from build123d import *

# Parameters (mm, degrees)
SKETCH1_R           = 18.5
BOSS_EXTRUDE1_DEPTH = 8.7
CUT_EXTRUDE1_START  = -5.7
SKETCH2_R           = 18.5
SKETCH2_R_2         = 17
CUT_EXTRUDE1_DEPTH  = 5.7
SKETCH3_R           = 14.2
CUT_EXTRUDE2_DEPTH  = 5.6
SKETCH4_R           = 4
BOSS_EXTRUDE2_DEPTH = 10
CHAMFER1_SIZE       = 2
SKETCH5_R           = 1.5
CUT_EXTRUDE3_DEPTH  = 30.259357478


with BuildPart() as part:
    # Sketch1 → Boss-Extrude1 (new body)
    with BuildSketch(Plane(origin=(0, 0, 0), x_dir=(1, 0, 0), z_dir=(0, 1, 0))):
        with Locations(Location((0, 0, 0), (0, 0, 270))):
            Circle(SKETCH1_R)
    extrude(amount=BOSS_EXTRUDE1_DEPTH)

    # Sketch2 → Cut-Extrude1 (cut)
    with BuildSketch(Plane(origin=(0, 8.7, 0), x_dir=(1, 0, 0), z_dir=(0, 1, 0)).offset(CUT_EXTRUDE1_START)):
        with Locations(Location((0, 0, 0), (0, 0, 270))):
            Circle(SKETCH2_R)
        with Locations(Location((0, 0, 0), (0, 0, 270))):
            Circle(SKETCH2_R_2, mode=Mode.SUBTRACT)
    extrude(amount=CUT_EXTRUDE1_DEPTH, mode=Mode.SUBTRACT)

    # Sketch3 → Cut-Extrude2 (cut)
    with BuildSketch(Plane.XZ):
        with Locations(Location((0, 0, 0), (0, 0, 270))):
            Circle(SKETCH3_R)
    extrude(amount=-CUT_EXTRUDE2_DEPTH, mode=Mode.SUBTRACT)

    # Sketch4 → Boss-Extrude2 (add)
    with BuildSketch(Plane(origin=(0, 8.7, 0), x_dir=(1, 0, 0), z_dir=(0, 1, 0))):
        with Locations(Location((0, 0, 0), (0, 0, 270))):
            Circle(SKETCH4_R)
    extrude(amount=BOSS_EXTRUDE2_DEPTH)

    # Chamfer1
    chamfer1_edges = [part.edges().sort_by_distance(p)[0] for p in [
        (0, 0, -18.5),
    ]]
    chamfer(chamfer1_edges, length=CHAMFER1_SIZE)

    # Sketch5 → Cut-Extrude3 (cut, through all)
    with BuildSketch(Plane.XZ.offset(-5.6)):
        with Locations(Location((0, 0, 0), (0, 0, 270))):
            Circle(SKETCH5_R)
    extrude(amount=-CUT_EXTRUDE3_DEPTH, mode=Mode.SUBTRACT)


solid = part.part
Part model, mm, in its own coordinate system. A direction names the side the tool comes from. Give positions to 0.01 mm unless a question says otherwise; leave off trailing zeros. Loops run counter-clockwise (first coordinate to the right, second up) from the corner with the lowest first, then second, coordinate; pieces in that order, holes last.
(1) 3-axis set-ups, long thin cutter, end or side, ignore diameter. For faces 4 (the cylindrical face through (11.973, 2.761, -7.634)), 5 (the flat face through (0, 18.7, 2)), 6 (the flat face through (-16.4, 3, 5.4)): which of +Z, -Z, +X, -X, +Y, -Y reach the whole face in a straight line?
Return value:
face 4: -Y
face 5: +Z, -Z, +X, -X, +Y
face 6: +Y
(2) Drill centre lines: line 1 along X through (y, z) = (2.45, 0); line 2 along Z through (x, y) = (-12, 3.5); line 3 along Z through (x, y) = (1, 2.25). Where is each one in solid material? Low to high.
Return value:
line 1: x = -18.5 to -14.2, 14.2 to 18.5
line 2: z = -12.04 to -7.59, 7.59 to 12.04
line 3: z = -18.47 to -14.16, 14.16 to 18.47
(3) Pin check, flat tips, straight feed: pin 1 (12 mm diameter, centred on x = 2.5, z = 2, fed in from -Y); pin 2 (1 mm diameter, centred on y = 6, z = 14.5, fed in from +X); pin 3 (10 mm diameter, centred on y = 8.5, z = 6.5, fed in from +X). Stop position of each tip, or through.
Return value:
pin 1: stops at y = 5.6
pin 2: stops at x = 9.64
pin 3: stops at x = 16.93
(4) Band-saw the part on B-B (x = 0). Write the cut outline in (y, z), and give its area (3 significant figures).
Return value:
outline: (0, -16.5) - (2, -18.5) - (3, -18.5) - (3, -17) - (8.7, -17) - (8.7, -4) - (18.7, -4) - (18.7, -1.5) - (5.6, -1.5) - (5.6, -14.2) - (0, -14.2) - close; (0, 14.2) - (5.6, 14.2) - (5.6, 1.5) - (18.7, 1.5) - (18.7, 4) - (8.7, 4) - (8.7, 17) - (3, 17) - (3, 18.5) - (2, 18.5) - (0, 16.5) - close
area: 182 mm2
(5) Band-saw the part on C-C (y = 8). Write the cut outline in (x, z).
Return value:
outline: circle Ø34 at (0, 0); hole circle Ø3 at (0, 0)
(6) Band-saw the part on A-A (z = 0). Write the cut outline in (x, y), and give its area (3 significant figures).
Return value:
outline: (-18.5, 2) - (-16.5, 0) - (-14.2, 0) - (-14.2, 5.6) - (-1.5, 5.6) - (-1.5, 18.7) - (-4, 18.7) - (-4, 8.7) - (-17, 8.7) - (-17, 3) - (-18.5, 3) - close; (1.5, 5.6) - (14.2, 5.6) - (14.2, 0) - (16.5, 0) - (18.5, 2) - (18.5, 3) - (17, 3) - (17, 8.7) - (4, 8.7) - (4, 18.7) - (1.5, 18.7) - close
area: 182 mm2
(7) Band-saw the part on D-D (y = 12.5). Write the cut outline in (x, z).
Return value:
outline: circle Ø8 at (0, 0); hole circle Ø3 at (0, 0)
(8) Pull direction X, two halves, no side cores. Call faces 1 (the flat face through (-3, 5.6, 0)), 2 (the flat face through (-4, 8.7, 4)), 3 (the cylindrical face through (-3.905, 13.63, -0.867)): pulls with the +X half, pulls with the -X half, needs draft (parallel to the pull), parting line crosses it, or undercut.
Return value:
face 1: undercut
face 2: needs draft
face 3: parting line crosses it
